```python
from build123d import *

# Parameters (mm, degrees)
SKETCH1_W          = 80
SKETCH1_H          = 84
SKETCH1_R          = 9.75
MAIN_BOSS_DEPTH    = 29
SKETCH2_R          = 28.5
CUT_EXTRUDE1_DEPTH = 17
FILLET1_R          = 15
SKETCH3_R          = 5.1
SCREW_HEAD_DEPTH   = 38
NUT_START          = -42
NUT_SLOT_DEPTH     = 4.8
SKETCH5_R          = 3.2
THROUGH_HOLE_DEPTH = 62
FILLET2_R          = 3
FILLET3_R          = 2
FILLET4_R          = 0.5


with BuildPart() as part:
    # Sketch1 → Main Boss (new body)
    with BuildSketch(Plane(origin=(0, 0, 0), x_dir=(0, 1, 0), z_dir=(0, 0, 1))):
        Rectangle(SKETCH1_W, SKETCH1_H)
        with Locations(Location((0, 0, 0), (0, 0, 90))):
            Circle(SKETCH1_R, mode=Mode.SUBTRACT)
    extrude(amount=MAIN_BOSS_DEPTH)

    # Sketch2 → Cut-Extrude1 (cut)
    with BuildSketch(Plane(origin=(0, 0, 0), x_dir=(1, 0, 0), z_dir=(0, 0, -1))):
        with Locations(Location((0, 0, 0), (0, 0, 180))):
            Circle(SKETCH2_R)
    extrude(amount=-CUT_EXTRUDE1_DEPTH, mode=Mode.SUBTRACT)

    # Fillet1
    # the kernel refuses this fillet: 15 mm, written as the material it takes off along each edge
    with BuildSketch(Plane(origin=(0, 0, 29), x_dir=(-1, 0, 0), z_dir=(0, 1, 0))) as fillet1_piece_1:
        with BuildLine():
            CenterArc((24.446938457, -15), FILLET1_R, 90, 78.463040967)
            Line((9.75, -12), (9.456061231, -11.94))
            ThreePointArc((9.456061231, -11.94), (9.45, -6), (9.45, 0))
            Line((9.45, 0), (9.75, 0.3))
            Line((9.75, 0.3), (24.446938457, 0.3))
            Line((24.446938457, 0.3), (24.446938457, 0))
        make_face()
    revolve(axis=Axis((0, 0, 29), (0, 0, 1)), mode=Mode.SUBTRACT)

    # Sketch3 → Screw Head (cut)
    with BuildSketch(Plane(origin=(0, 40, 0), x_dir=(-1, 0, 0), z_dir=(0, 1, 0))):
        with Locations((-35.025, 14.5)):
            Circle(SKETCH3_R)
        with Locations((35.025, 14.5)):
            Circle(SKETCH3_R)
    extrude(amount=-SCREW_HEAD_DEPTH, mode=Mode.SUBTRACT)

    # Sketch4 → Nut Slot (cut)
    with BuildSketch(Plane(origin=(0, 40, 0), x_dir=(-1, 0, 0), z_dir=(0, 1, 0)).offset(NUT_START)):
        Polygon((-30.324429276, 17.852307892), (-35.577898433, 20.246967605), (-40.278469158, 16.894659714), (-39.725570724, 11.147692108), (-34.472101567, 8.753032395), (-29.771530842, 12.105340286), align=None)
    nut_slot = extrude(amount=-NUT_SLOT_DEPTH, mode=Mode.SUBTRACT)

    # Sketch5 → Through Hole (cut)
    with BuildSketch(Plane(origin=(0, 40, 0), x_dir=(-1, 0, 0), z_dir=(0, 1, 0))):
        with Locations((-35.025, 14.5)):
            Circle(SKETCH5_R)
    through_hole = extrude(amount=-THROUGH_HOLE_DEPTH, mode=Mode.SUBTRACT)

    # Mirror2: Nut Slot, Through Hole across plane
    add(nut_slot.mirror(Plane(origin=(0, 0, 0), x_dir=(0, 0, 1), z_dir=(1, 0, 0))), mode=Mode.SUBTRACT)
    add(through_hole.mirror(Plane(origin=(0, 0, 0), x_dir=(0, 0, 1), z_dir=(1, 0, 0))), mode=Mode.SUBTRACT)

    # Fillet2
    fillet2_edges = [part.edges().sort_by_distance(p)[0] for p in [
        (28.5, 0, 17),
    ]]
    fillet(fillet2_edges, radius=FILLET2_R)

    # Fillet3
    # the kernel refuses this fillet: 2 mm, written as the material it takes off along each edge
    with BuildSketch(Plane(origin=(42, 40, -5), x_dir=(0, -1, 0), z_dir=(0, 0, 1)), Plane(origin=(-42, 40, -5), x_dir=(1, 0, 0), z_dir=(0, 0, 1))) as fillet3_piece_1:
        with BuildLine():
            CenterArc((FILLET3_R, -FILLET3_R), FILLET3_R, 90, 90)
            Line((0, -FILLET3_R), (0, 0))
            Line((0, 0), (FILLET3_R, 0))
        make_face()
    extrude(amount=39, mode=Mode.SUBTRACT)
    with BuildSketch(Plane(origin=(42, -40, -5), x_dir=(0, 1, 0), z_dir=(0, 0, 1)), Plane(origin=(-42, -40, -5), x_dir=(1, 0, 0), z_dir=(0, 0, 1))) as fillet3_piece_2:
        with BuildLine():
            CenterArc((FILLET3_R, FILLET3_R), FILLET3_R, 180, 90)
            Line((0, FILLET3_R), (0, 0))
            Line((0, 0), (FILLET3_R, 0))
        make_face()
    extrude(amount=39, mode=Mode.SUBTRACT)

    # Fillet4
    fillet4_edges = [part.edges().sort_by_distance(p)[0] for p in [
        (34.46042051, 40, 19.568653667),
        (-40.093653599, 39.997806015, 15.064580313),
        (40.125, 39.996089928, 14.5),
        (-29.925, 40, 14.5),
    ]]
    fillet(fillet4_edges, radius=FILLET4_R)


solid = part.part
```
The listing builds one solid part. Answer for the finished solid, in the listing's coordinates (mm). A direction names the side the tool comes from. Give positions to 0.01 mm unless a question says otherwise; leave off trailing zeros. Order: outer loops, then holes, each group sorted by start corner. A loop starts at its lowest first (then second) coordinate and runs counter-clockwise, first axis right, second up. Notation, with made-up numbers: (76, 9) - (85, 9) arc R35 cw to (85, 43) - close; hole circle Ø7 at (-33.5, 11.25). An arc over 180 degrees is marked (long way). Use one line per item in the form item = value. Start each with the question number.
(1) The mould has two halves that part along Y. Classify faces 4 (the flat face through (32.91, -4.37, 19.03)), 5 (the cylindrical face through (37.6, 0, 12.6)), 6 (the flat face through (35, 2, 11)): released by +Y, released by -Y, zero draft, split by the parting line, or undercut.
(2) Flat-ended cylindrical pins translate along their axes: pin 1 Ø6 at (x, z) = (-35.025, 14.5) entering from +Y; pin 2 Ø7 at (x, z) = (-35, 15) entering from +Y. Find the tip coordinate at first contact, or state that the pin passes through.
(3) For faces 1 (the cylindrical face through (-41.4, 39.43, 14.3)), 2 (the flat face through (-37.4, -6.8, 17.1)), 3 (the flat face through (-38.4, 2, 14.6)), determine the directions among +Z, -Z, +X, -X, +Y, -Y from which every point of the face is accessible in a straight line to the end or side of a thin tool.
(4) Consider line 1 (Y direction, x = 0, z = 11); line 2 (X direction, y = -21.5, z = 13); line 3 (Y direction, x = 34, z = 18). Determine where each line is inside the solid, lowest interval first. Write a range as from..to.
(5) A cutting plane is placed at C-C, the plane z = 27. Write down the section's boundary in (x, y), then the cut area to 3 significant figures.
(6) A cutting plane is placed at B-B, the plane x = 0. Write down the section's boundary in (y, z).
(7) A cutting plane is placed at A-A, the plane y = 0. Write down the section's boundary in (x, z) (3 decimals), then the cut area to 3 significant figures.
(8) A cutting plane is placed at D-D, the plane y = 32. Write down the section's boundary in (x, z) (3 decimals).
Ans:
q1.face_4 = undercut
q1.face_5 = zero draft
q1.face_6 = released by +Y
q2.pin_1 = -22
q2.pin_2 = 2
q3.face_1 = +Z, -Z, -X, +Y
q3.face_2 = none
q3.face_3 = +Y
q4.line_1 = -40..-28.5, 28.5..40
q4.line_2 = -42..-37.85, -32.2..-18.71, 18.71..32.2, 37.85..42
q4.line_3 = -40..-6.8, -2..2
q5.outline = (-42, -38) arc R2 ccw to (-40, -40) - (40, -40) arc R2 ccw to (42, -38) - (42, 38) arc R2 ccw to (40, 40) - (-40, 40) arc R2 ccw to (-42, 38) - close; hole circle Ø33.93 at (0, 0)
q5.area = 5,810 mm^2
q6.outline = (-40, 0) - (-28.5, 0) - (-28.5, 14) arc R3 cw to (-25.5, 17) - (-9.75, 17) arc R15 ccw to (-24.45, 29) - (-40, 29) - close; (9.75, 17) - (25.5, 17) arc R3 cw to (28.5, 14) - (28.5, 0) - (40, 0) - (40, 29) - (24.45, 29) arc R15 ccw to start
q7.outline = (-42, 0) - (-28.5, 0) - (-28.5, 14) arc R3 cw to (-25.5, 17) - (-9.75, 17) arc R15 ccw to (-24.447, 29) - (-42, 29) - close; (9.75, 17) - (25.5, 17) arc R3 cw to (28.5, 14) - (28.5, 0) - (42, 0) - (42, 29) - (24.447, 29) arc R15 ccw to start; hole circle Ø6.4 at (-35.025, 14.5); hole circle Ø6.4 at (35.025, 14.5)
q7.area = 1,080 mm^2
q8.outline = (-42, 0) - (42, 0) - (42, 29) - (-42, 29) - close; hole circle Ø10.2 at (-35.025, 14.5); hole circle Ø10.2 at (35.025, 14.5)
